Build history of the part. All positions in model axes, mm. A direction names the side the tool comes from. Give positions to 0.01 mm unless a question says otherwise; leave off trailing zeros. Order: outer loops, then holes, each group sorted by start corner. A loop starts at its lowest first (then second) coordinate and runs counter-clockwise, first axis right, second up. Notation, with made-up numbers: M 1,55 L 14,55 A19 cw 14,60 Z; hole C -9,27 d4. An arc over 180 degrees is marked long. One line per item, written item: value.
from build123d import *
from build123d import SkipClean  # not in build123d's __all__

# Parameters (mm, degrees)
F0_R      = 1.65
F1_DEPTH  = 1.5
F3_DEPTH  = 1.501
F4_DEPTH  = 1.5
F5_W      = 40
F5_H      = 30
F6_DEPTH  = 3
F7_W      = 36
F7_H      = 23.3
F8_DEPTH  = 9
F10_DEPTH = 1.501


with BuildPart() as f1:
    # F0 (on Top) → F1 (new body)
    with BuildSketch(Plane.XY):
        with BuildLine():
            ThreePointArc((-0.73370891, 14), (-0.4891889552, 6.9935887205), (0, 0))
            Line((0, 0), (65, 0))
            ThreePointArc((65, 0), (65.4891889552, 6.9935887205), (65.73370891, 14))
            ThreePointArc((65.73370891, 14), (65.7334108185, 21.0021379582), (65.488741818, 28))
            Line((65.488741818, 28), (57.299411547, 50.5))
            ThreePointArc((57.299411547, 50.5), (32.5, 63.5), (7.700588453, 50.5))
            Line((7.700588453, 50.5), (-0.488741818, 28))
            ThreePointArc((-0.488741818, 28), (-0.7334108185, 21.0021379582), (-0.73370891, 14))
        make_face()
        with Locations((4.5, 12.5)):
            Circle(F0_R, mode=Mode.SUBTRACT)
        with Locations((60.5, 12.5)):
            Circle(F0_R, mode=Mode.SUBTRACT)
        with Locations((15, 54.5)):
            Circle(F0_R, mode=Mode.SUBTRACT)
    extrude(amount=F1_DEPTH)

    # F2 (on face) → F3 (cut, through all)
    with BuildSketch(Plane.XY.offset(1.5)):
        with BuildLine():
            ThreePointArc((15.3946260476, 58.178895253), (17.4713893755, 57.2535857631), (18.6149922575, 55.2885626028))
            Line((18.6149922575, 55.2885626028), (20.0740134556, 48.6))
            Line((20.0740134556, 48.6), (52.5, 48.6))
            Line((52.5, 48.6), (52.5, 24.064025175))
            Line((52.5, 24.064025175), (62.8817094627, 15.3315119698))
            ThreePointArc((62.8817094627, 15.3315119698), (63.8542752579, 14.0616777817), (64.2, 12.5))
            ThreePointArc((64.2, 12.5), (62.0616777817, 9.1457247421), (58.1182905373, 9.6684880302))
            Line((58.1182905373, 9.6684880302), (47.5, 18.6))
            Line((47.5, 18.6), (17.5, 18.6))
            Line((17.5, 18.6), (6.8817094627, 9.6684880302))
            ThreePointArc((6.8817094627, 9.6684880302), (1.6684880302, 10.1182905373), (2.1182905373, 15.3315119698))
            Line((2.1182905373, 15.3315119698), (12.5, 24.064025175))
            Line((12.5, 24.064025175), (12.5, 48.6))
            Line((12.5, 48.6), (11.3850077425, 53.7114373972))
            ThreePointArc((11.3850077425, 53.7114373972), (11.308192582, 54.2539146721), (11.3123280961, 54.8017878876))
            ThreePointArc((11.3123280961, 54.8017878876), (9.4060764304, 52.7351735725), (7.700588453, 50.5))
            Line((7.700588453, 50.5), (-0.488741818, 28))
            ThreePointArc((-0.488741818, 28), (-0.733560046, 13.9914611719), (0, 0))
            Line((0, 0), (65, 0))
            ThreePointArc((65, 0), (65.733560046, 13.9914611719), (65.488741818, 28))
            Line((65.488741818, 28), (57.299411547, 50.5))
            ThreePointArc((57.299411547, 50.5), (37.9351551683, 63.0061258111), (15.3946260476, 58.178895253))
        make_face()
    extrude(amount=-F3_DEPTH, mode=Mode.SUBTRACT)

    # F2 (on face) → F4 (join)
    with BuildSketch(Plane.XY.offset(1.5)):
        with BuildLine():
            ThreePointArc((11.3123280961, 54.8017878876), (13.2791635515, 56.5801728664), (15.3946260476, 58.178895253))
            ThreePointArc((15.3946260476, 58.178895253), (12.6415574435, 57.3509206772), (11.3123280961, 54.8017878876))
        make_face()
    with SkipClean():  # cleaning this boolean's faces spoils the solid; the shape is the same uncleaned
        extrude(amount=-F4_DEPTH)

    # F5 (on face) → F6 (join)
    with BuildSketch(Plane.XY.offset(1.5)):
        with Locations((32.5, 33.6)):
            Rectangle(F5_W, F5_H)
    extrude(amount=F6_DEPTH)

    # F7 (on face) → F8 (join)
    with BuildSketch(Plane.XY.offset(4.5)):
        with Locations((32.5, 30.25)):
            Rectangle(F7_W, F7_H)
    extrude(amount=F8_DEPTH)

    # F9 (on face) → F10 (cut, through all)
    with BuildSketch(Plane.XY.offset(1.5)):
        with BuildLine():
            ThreePointArc((7.348777143, 10.0613592332), (8.0174859123, 11.2000796728), (8.25, 12.5))
            ThreePointArc((8.25, 12.5), (6.3550732217, 15.7590187699), (2.5853582175, 15.7243831727))
            ThreePointArc((2.5853582175, 15.7243831727), (1.6302243549, 10.0861052742), (7.348777143, 10.0613592332))
        make_face()
        with BuildLine():
            ThreePointArc((2.5853582175, 15.7243831727), (6.3550732217, 15.7590187699), (8.25, 12.5))
            ThreePointArc((8.25, 12.5), (8.0174859123, 11.2000796728), (7.348777143, 10.0613592332))
            Line((7.348777143, 10.0613592332), (17.5, 18.6))
            Line((17.5, 18.6), (12.5, 18.6))
            Line((12.5, 18.6), (12.5, 24.064025175))
            Line((12.5, 24.064025175), (2.5853582175, 15.7243831727))
        make_face()
    extrude(amount=-F10_DEPTH, mode=Mode.SUBTRACT)


solid = f1.part
1) Tool access for faces 5 (the face through (12.5, 33, 2)), 6 (the face through (16, 52, 1.5)), 7 (the face through (50.5, 30, 9)), 8 (the face through (14.5, 30, 9)): list every direction of +Z, -Z, +X, -X, +Y, -Y with a clear straight run to the whole face (end or side of a thin tool).
Check values:
face 5: +Z, -Z, -X, -Y
face 6: +Z, +X, -X, +Y
face 7: +Z, +X, +Y, -Y
face 8: +Z, -X, +Y, -Y
2) Saw through at A-A, the plane y = 33. Write the cut outline in (x, z).
Check values:
outline: M 12.5,0 L 52.5,0 L 52.5,4.5 L 50.5,4.5 L 50.5,13.5 L 14.5,13.5 L 14.5,4.5 L 12.5,4.5 Z
3) Saw through at D-D, the plane z = 10.25. Write the cut outline in (x, y).
Check values:
outline: M 14.5,18.6 L 50.5,18.6 L 50.5,41.9 L 14.5,41.9 Z
4) Saw through at B-B, the plane x = 60.5. Write the cut outline in (y, z).
Check values:
outline: M 8.8,0 L 10.85,0 L 10.85,1.5 L 8.8,1.5 Z; M 14.15,0 L 17.33,0 L 17.33,1.5 L 14.15,1.5 Z
5) Mould opens along X. For faces 1 (the face through (16.574, 54.996, 0.74)), 2 (the face through (58.85, 12.57, 0.74)), 3 (the face through (31, 43, 4.5)), 4 (the face through (52.883, 14.072, 0.76)) say: released by +X, released by -X, zero draft, split by the parting line, or undercut.
Check values:
face 1: undercut
face 2: undercut
face 3: zero draft
face 4: released by -X
6) Saw through at C-C, the plane z = 2.5. Write the cut outline in (x, y), then the cut area to 3 significant figures.
Check values:
outline: M 12.5,18.6 L 52.5,18.6 L 52.5,48.6 L 12.5,48.6 Z
area: 1,200 mm^2
7) Pin check, flat tips, straight feed: pin 1 (1 mm diameter, centred on x = 50, z = 4, fed in from -Y); pin 2 (10 mm diameter, centred on x = 29.5, y = 43.5, fed in from +Z); pin 3 (1.3 mm diameter, centred on y = 38.5, z = 1, fed in from -X); pin 4 (7 mm diameter, centred on x = 36, z = 7.5, fed in from +Y). Stop position of each tip, or through.
Check values:
pin 1: y = 18.6
pin 2: z = 13.5
pin 3: x = 12.5
pin 4: y = 48.6
8) Drill centre lines: probe 1 along Y at (x, z) = (15, 0.65); probe 2 along Y at (x, z) = (60.5, 0.9); probe 3 along Z at (x, y) = (53, 17). Where is each one in solid material? Low to high. Write a range as from..to.
Check values:
probe 1: 18.6..52.85, 56.15..58.2
probe 2: 8.8..10.85, 14.15..17.33
probe 3: 0..1.5
